Source: CAD feature listing. Evaluate the final solid. Frame: model axes, mm. A direction names the side the tool comes from. Give positions to 0.01 mm unless a question says otherwise; leave off trailing zeros. Order: outer loops, then holes, each group sorted by start corner. A loop starts at its lowest first (then second) coordinate and runs counter-clockwise, first axis right, second up. Notation, with made-up numbers: M -36.5,73 L -27.5,73 A26 cw -27.5,96 Z; hole C 28.25,66.5 d9. An arc over 180 degrees is marked long. One line per question, with ' | ' between items. Start each with the question number.
from build123d import *

# Parameters (mm, degrees)
F0_W     = 304.8
F0_H     = 254
F1_DEPTH = 25.4
F2_R     = 3.96875
F3_DEPTH = 25.4
F4_R     = 9.525
F4_R_2   = 3.96875
F5_DEPTH = 9.525
F2_R_2   = 7.9375
F6_DEPTH = 25.4


with BuildPart() as f1:
    # F0 (on Top) → F1 (new body)
    with BuildSketch(Plane.XY):
        with Locations((152.4, 127)):
            Rectangle(F0_W, F0_H)
    extrude(amount=-F1_DEPTH)

    # F2 (on face) → F3 (cut)
    with BuildSketch(Plane.XY):
        with Locations((107.95, 171.45)):
            Circle(F2_R)
        with Locations((196.85, 171.45)):
            Circle(F2_R)
        with Locations((196.85, 82.55)):
            Circle(F2_R)
        with Locations((107.95, 82.55)):
            Circle(F2_R)
    extrude(amount=-F3_DEPTH, mode=Mode.SUBTRACT)

    # F4 (on face) → F5 (cut)
    with BuildSketch(Plane(origin=(0, 0, -25.4), x_dir=(1, 0, 0), z_dir=(0, 0, -1))):
        with Locations((107.95, -171.45)):
            Circle(F4_R)
        with Locations((107.95, -171.45)):
            Circle(F4_R_2, mode=Mode.SUBTRACT)
        with Locations((196.85, -171.45)):
            Circle(F4_R)
        with Locations((196.85, -171.45)):
            Circle(F4_R_2, mode=Mode.SUBTRACT)
        with Locations((107.95, -82.55)):
            Circle(F4_R)
        with Locations((107.95, -82.55)):
            Circle(F4_R_2, mode=Mode.SUBTRACT)
        with Locations((196.85, -82.55)):
            Circle(F4_R)
        with Locations((196.85, -82.55)):
            Circle(F4_R_2, mode=Mode.SUBTRACT)
    extrude(amount=-F5_DEPTH, mode=Mode.SUBTRACT)

    # F2 (on face) → F6 (cut)
    with BuildSketch(Plane.XY):
        with Locations((107.95, 171.45)):
            Circle(F2_R)
        with Locations((196.85, 171.45)):
            Circle(F2_R)
        with Locations((107.95, 82.55)):
            Circle(F2_R)
        with Locations((196.85, 82.55)):
            Circle(F2_R)
        with Locations((25.4, 215.9)):
            Circle(F2_R_2)
        with Locations((279.4, 215.9)):
            Circle(F2_R_2)
        with Locations((279.4, 38.1)):
            Circle(F2_R_2)
        with Locations((25.4, 38.1)):
            Circle(F2_R_2)
    extrude(amount=-F6_DEPTH, mode=Mode.SUBTRACT)


solid = f1.part
Item 1: Cut plane D-D on x = 25.4. Return the cut outline in (y, z), and give its area (3 significant figures).
Item 2: Cut plane B-B on y = 171.45. Return the cut outline in (x, z) (3 decimals), and give its area (3 significant figures).
Item 3: Cut plane C-C on z = -20. Count the separate pieces of the cut face and the enclosed holes in it, and give its area (3 significant figures).
Item 4: Line query: line 1 (Y direction, x = 107.95, z = -6.5); line 2 (X direction, y = 216, z = -11); line 3 (Y direction, x = 107.95, z = -19.5) (3 decimals). Output: solid intervals per line, ascending.
Item 5: Reachability of faces 4 (the cylindrical face through (205.65, 86.2, -20.7)), 5 (the flat face through (150, 129, 0)) from +Z, -Z, +X, -X, +Y, -Y: full face, straight path, thin tool, end or side. Return the list, or none.
Item 6: Cut plane A-A on x = 107.95. Return the cut outline in (y, z) (3 decimals), and give its area (3 significant figures).
Item 7: Mould query, pull axis Y, two halves, no side actions, for faces 1 (the flat face through (0, 125, -13)), 2 (the flat face through (150, 0, -13)), 3 (the flat face through (108, 176, -15.875)). Classes: pulls with the +Y half, pulls with the -Y half, needs draft (parallel to the pull), parting line crosses it, or undercut.
Item 8: Pin query (flat end, axial travel): pin 1 Ø9 at (x, y) = (107.95, 82.55) entering from -Z (3 decimals). Return the tip coordinate at first contact, or that it passes through.
Results are:
1) outline: M 0,-25.4 L 30.16,-25.4 L 30.16,0 L 0,0 Z; M 46.04,-25.4 L 207.96,-25.4 L 207.96,0 L 46.04,0 Z; M 223.84,-25.4 L 254,-25.4 L 254,0 L 223.84,0 Z | area: 5,650 mm2
2) outline: M 0,-25.4 L 98.425,-25.4 L 98.425,-15.875 L 103.981,-15.875 L 103.981,0 L 0,0 Z; M 111.919,-15.875 L 117.475,-15.875 L 117.475,-25.4 L 187.325,-25.4 L 187.325,-15.875 L 192.881,-15.875 L 192.881,0 L 111.919,0 Z; M 200.819,-15.875 L 206.375,-15.875 L 206.375,-25.4 L 304.8,-25.4 L 304.8,0 L 200.819,0 Z | area: 7,130 mm2
3) separate pieces: 1 | enclosed holes: 8 | area: 75,500 mm2
4) line 1: y = 0 to 78.58, 86.52 to 167.48, 175.42 to 254 | line 2: x = 0 to 17.46, 33.34 to 271.46, 287.34 to 304.8 | line 3: y = 0 to 73.025, 92.075 to 161.925, 180.975 to 254
5) face 4: -Z | face 5: +Z, +X, -X, +Y, -Y
6) outline: M 0,-25.4 L 73.025,-25.4 L 73.025,-15.875 L 78.581,-15.875 L 78.581,0 L 0,0 Z; M 86.519,-15.875 L 92.075,-15.875 L 92.075,-25.4 L 161.925,-25.4 L 161.925,-15.875 L 167.481,-15.875 L 167.481,0 L 86.519,0 Z; M 175.419,-15.875 L 180.975,-15.875 L 180.975,-25.4 L 254,-25.4 L 254,0 L 175.419,0 Z | area: 5,840 mm2
7) face 1: needs draft | face 2: pulls with the -Y half | face 3: undercut
8) pin 1: stops at z = -15.875
